from build123d import *

# Parameters (mm, degrees)
F0_W     = 50.8
F0_H     = 50.8
F1_DEPTH = 50.8
F3_R     = 5.08
F5_T     = -2.54
F7_D     = 6.35


# Not quite as in the source:
# - a shell that OpenCascade refuses in one call is made with other operations: the cavity is built on its own and cut out


with BuildPart() as f1:
    # F0 (on Top) → F1 (new body)
    with BuildSketch(Plane.XY):
        with Locations((-29.015717721, -32.2184429228)):
            Rectangle(F0_W, F0_H)
    extrude(amount=F1_DEPTH)

    # F3
    f3_edges = [f1.edges().sort_by_distance(p)[0] for p in [
        (-29.015718, -57.618443, 50.8),
        (-54.415718, -32.218443, 50.8),
        (-29.015718, -6.818443, 50.8),
        (-3.615718, -32.218443, 50.8),
        (-54.415718, -57.618443, 25.4),
        (-54.415718, -6.818443, 25.4),
        (-3.615718, -6.818443, 25.4),
        (-3.615718, -57.618443, 25.4),
        (-3.615718, -32.218443, 0),
    ]]
    fillet(f3_edges, radius=F3_R)

    # F5: a shell. OpenCascade refuses it in one call, so the cavity is built on its own and cut out:
    # the body offset inwards by the wall thickness, plus a prism from it out through each open face.
    f5_core = offset(f1.part, amount=F5_T, mode=Mode.PRIVATE)
    f5_exits = [f5_core.faces().sort_by_distance(p)[0] for p in [
        (-6.155718, -32.218443, 25.4),
    ]]
    add(f5_core, mode=Mode.SUBTRACT)
    extrude(f5_exits, amount=-F5_T, mode=Mode.SUBTRACT)

    # F7 (through all)
    with Locations(Plane.XY.offset(50.8)):
        with Locations((-29.1464701295, -31.9354347885)):
            Hole(F7_D / 2)


solid = f1.part
Geometry: final body of the model. Coordinates: model frame, mm. A direction names the side the tool comes from. Round coordinates to 2 decimals unless told otherwise and drop trailing zeros. Loops run counter-clockwise (first coordinate to the right, second up) from the corner with the lowest first, then second, coordinate; pieces in that order, holes last.
Q1. Section B-B on z = 10.5. Return loops of the section in (x, y), plus the area to 3 significant figures.
Q2. Pull-direction query (X, two-part tool) for faces 1 (the cylindrical face through (-51.151, -54.315, 24.432)), 2 (the cylindrical face through (-52.97, -56.09, 23.18)), 3 (the flat face through (-5, -33, 5.08)); classes: released by +X, released by -X, zero draft, split by the parting line, or undercut.
Q3. Section D-D on x = -29.5. Return loops of the section in (y, z).
Q4. Pin query (flat end, axial travel): P1, Ø10, axis at y = -26, z = 8.5, coming from the +X side; P2, Ø3, axis at x = -4.5, z = 24, coming from the -Y side; P3, Ø5.5, axis at x = -29.15, y = -31.94, coming from the +Z side; P4, Ø0.8, axis at x = -5, y = -24, coming from the -Z side. Return the tip coordinate at first contact, or that it passes through.
Q5. Access query for faces 4 (the cylindrical face through (-6.92, -54.354, 24.432)), 5 (the flat face through (-5, -52.538, 25)), 6 (the flat face through (-37, -32, 0)). Directions: +Z, -Z, +X, -X, +Y, -Y. A direction counts if a zero-diameter tool reaches every point of the face in a straight line with its end or side. Return the directions, or none.
Q6. Section A-A on x = -43.5. Return loops of the section in (y, z).
Q7. Material intervals for L1, parallel to Y at x = -17.5, z = 45; L2, parallel to Z at x = -30, y = -20; L3, parallel to X at y = -42.5, z = 24, sorted ascending.
Q8. Section C-C on y = -42.5. Return loops of the section in (x, z).
Evaluation:
1. outline: (-54.42, -52.54) arc R5.08 ccw to (-49.34, -57.62) - (-8.7, -57.62) arc R5.08 ccw to (-3.62, -52.54) - (-6.16, -52.54) arc R2.54 cw to (-8.7, -55.08) - (-49.34, -55.08) arc R2.54 cw to (-51.88, -52.54) - (-51.88, -11.9) arc R2.54 cw to (-49.34, -9.36) - (-8.7, -9.36) arc R2.54 cw to (-6.16, -11.9) - (-3.62, -11.9) arc R5.08 ccw to (-8.7, -6.82) - (-49.34, -6.82) arc R5.08 ccw to (-54.42, -11.9) - close
1. area: 370 mm2
2. face 1: undercut
2. face 2: released by -X
2. face 3: zero draft
3. outline: (-57.62, 0) - (-35.09, 0) - (-35.09, 2.54) - (-55.08, 2.54) - (-55.08, 45.72) arc R2.54 cw to (-52.54, 48.26) - (-35.09, 48.26) - (-35.09, 50.8) - (-52.54, 50.8) arc R5.08 ccw to (-57.62, 45.72) - close; (-28.78, 0) - (-6.82, 0) - (-6.82, 45.72) arc R5.08 ccw to (-11.9, 50.8) - (-28.78, 50.8) - (-28.78, 48.26) - (-11.9, 48.26) arc R2.54 cw to (-9.36, 45.72) - (-9.36, 2.54) - (-28.78, 2.54) - close
4. P1: stops at x = -3.62
4. P2: stops at y = -56.84
4. P3: passes through
4. P4: stops at z = 1.21
5. face 4: none
5. face 5: +X
5. face 6: -Z, +X, -X, +Y, -Y
6. outline: (-57.62, 0) - (-6.82, 0) - (-6.82, 45.72) arc R5.08 ccw to (-11.9, 50.8) - (-52.54, 50.8) arc R5.08 ccw to (-57.62, 45.72) - close; hole (-55.08, 2.54) - (-9.36, 2.54) - (-9.36, 45.72) arc R2.54 ccw to (-11.9, 48.26) - (-52.54, 48.26) arc R2.54 ccw to (-55.08, 45.72) - close
7. L1: y = -57.62 to -55.08, -9.36 to -6.82
7. L2: z = 0 to 2.54, 48.26 to 50.8
7. L3: x = -54.42 to -51.88
8. outline: (-54.42, 0) - (-8.7, 0) arc R5.08 ccw to (-3.62, 5.08) - (-6.16, 5.08) arc R2.54 cw to (-8.7, 2.54) - (-51.88, 2.54) - (-51.88, 45.72) arc R2.54 cw to (-49.34, 48.26) - (-8.7, 48.26) arc R2.54 cw to (-6.16, 45.72) - (-3.62, 45.72) arc R5.08 ccw to (-8.7, 50.8) - (-49.34, 50.8) arc R5.08 ccw to (-54.42, 45.72) - close
